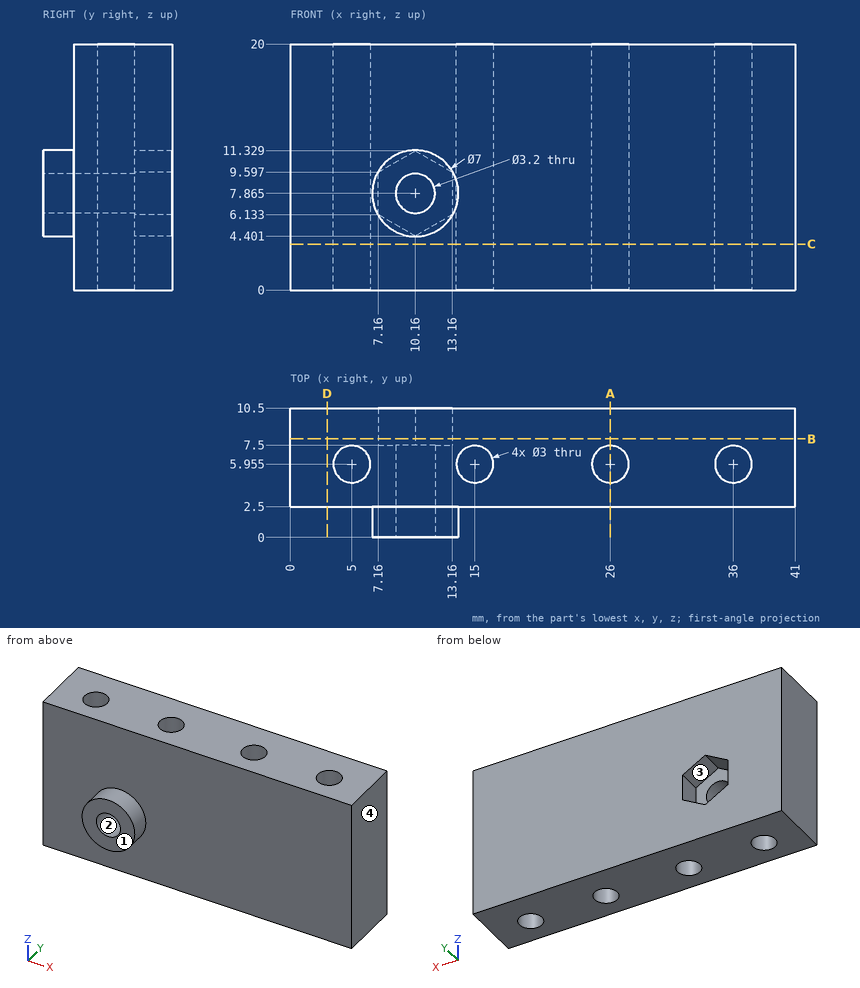
The drawing under review shows one solid part. Ordinate dimensions are in mm from its lowest x, y, z. Coordinates: 2 decimals unless noted, no trailing zeros. Write each loop counter-clockwise with the first axis right and the second up, starting at its lowest first coordinate (ties: lowest second). Pieces come first, ordered by that corner, then holes.
1) Add section C-C (z = 3.75). Write out the cut boundary in (x, y) (3 decimals), plus the area to 3 significant figures.
2) Add section D-D (x = 3). Write out the cut boundary in (y, z), plus the area to 3 significant figures.
3) Insertion check: pin 1 (5 mm diameter, centred on x = 20.5, y = 6, fed in from -Z); pin 2 (1.5 mm diameter, centred on x = 19, z = 12, fed in from -Y); pin 3 (5 mm diameter, centred on x = 10.16, z = 7.865, fed in from +Y). Each pin has a flat end and moves straight along its axis. Give the tip position at first contact, or say it passes through.
4) Mouldability with a two-part tool opening along X and no side actions: class the marked faces 1, 2, 3 and 4 as +X half, -X half, draft (parallel to the pull), parting line (faces both ways), or undercut.
5) Add section A-A (x = 26). Write out the cut boundary in (y, z) (3 decimals).
6) Add section B-B (y = 8). Write out the cut boundary in (x, z), plus the area to 3 significant figures.
7) To check wall thickness, follow L1, parallel to Y at x = 5, z = 15 (3 decimals); L2, parallel to X at y = 6, z = 7.5; L3, parallel to X at y = 4.75, z = 3.25. State the ranges of each line that lie inside material, in increasing order.
Check result:
1. outline: (0, 2.5) - (41, 2.5) - (41, 10.5) - (0, 10.5) - close; hole circle Ø3 at (5, 5.955); hole circle Ø3 at (15, 5.955); hole circle Ø3 at (26, 5.955); hole circle Ø3 at (36, 5.955)
1. area: 300 mm2
2. outline: (2.5, 0) - (10.5, 0) - (10.5, 20) - (2.5, 20) - close
2. area: 160 mm2
3. pin 1: stops at z = 0
3. pin 2: stops at y = 2.5
3. pin 3: stops at y = 7.5
4. face 1: draft
4. face 2: undercut
4. face 3: undercut
4. face 4: +X half
5. outline: (2.5, 0) - (4.455, 0) - (4.455, 20) - (2.5, 20) - close; (7.455, 0) - (10.5, 0) - (10.5, 20) - (7.455, 20) - close
6. outline: (0, 0) - (41, 0) - (41, 20) - (0, 20) - close; hole (7.16, 6.13) - (10.16, 4.4) - (13.16, 6.13) - (13.16, 9.6) - (10.16, 11.33) - (7.16, 9.6) - close
6. area: 789 mm2
7. L1: y = 2.5 to 4.455, 7.455 to 10.5
7. L2: x = 0 to 3.5, 6.5 to 8.6, 11.72 to 13.5, 16.5 to 24.5, 27.5 to 34.5, 37.5 to 41
7. L3: x = 0 to 4.11, 5.89 to 14.11, 15.89 to 25.11, 26.89 to 35.11, 36.89 to 41
